The drawing under review shows one solid part. Ordinate dimensions are in mm from its lowest x, y, z. A direction names the side the tool comes from. Coordinates: 2 decimals unless noted, no trailing zeros. Write each loop counter-clockwise with the first axis right and the second up, starting at its lowest first coordinate (ties: lowest second). Pieces come first, ordered by that corner, then holes. Notation, with made-up numbers: M -20.75,69.25 L -9.75,69.25 A22 ccw -9.75,78.25 Z; hole C 49.5,75.25 d1. An arc over 180 degrees is marked long. Write item = value, one per line.
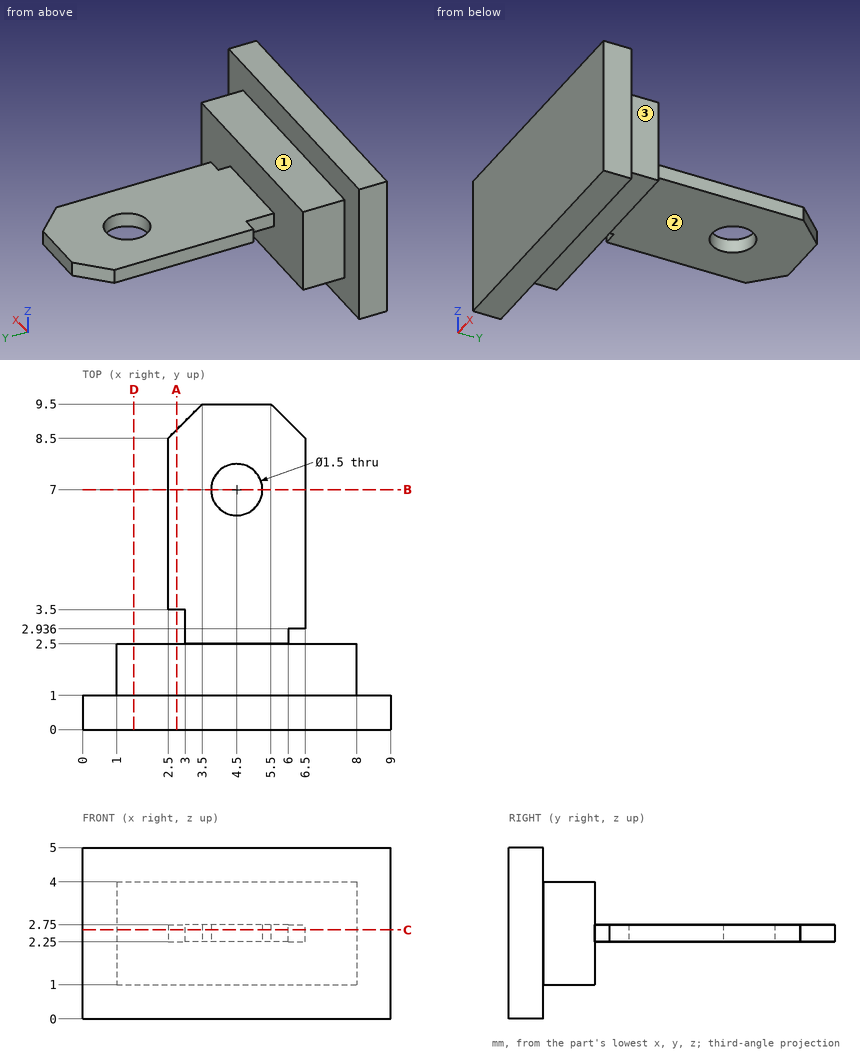
Q1. For P1, Ø4, axis at x = 7.5, y = 3.5, coming from the +Z side; P2, Ø1.2, axis at y = 2, z = 2, coming from the +X side; P3, Ø1.6, axis at x = 6, y = 2, coming from the -Z side, all flat-tipped, find the tip position at first contact; note any pin that passes through.
Check result:
P1 = 4
P2 = 8
P3 = 1
Q2. Consider section A-A, the plane x = 2.75. State the section outline as (y, z) points.
Check result:
outline = M 0,0 L 1,0 L 1,1 L 2.5,1 L 2.5,4 L 1,4 L 1,5 L 0,5 Z; M 3.5,2.25 L 8.75,2.25 L 8.75,2.75 L 3.5,2.75 Z
Q3. Wall thickness on line 1 (Y direction, x = 4.5, z = 2.45); line 2 (Y direction, x = 7.75, z = 0.75); line 3 (Y direction, x = 3, z = 3.4): over which ranges is each line inside the solid? List them lowest first.
Check result:
line_1 = 0 to 6.25, 7.75 to 9.5
line_2 = 0 to 1
line_3 = 0 to 2.5
Q4. Machinability: for the marked faces 1, 2 and 3, which of the approach directions +Z, -Z, +X, -X, +Y, -Y give a long, thin tool a straight path to every point of the face, cutting with its end or side? Answer none if there is none.
Check result:
face_1 = +Z, +X, -X, +Y
face_2 = -Z, +X, -X, +Y
face_3 = +Z, -Z, +X, +Y
Q5. Consider section D-D, the plane x = 1.5. State the section outline as (y, z) points.
Check result:
outline = M 0,0 L 1,0 L 1,1 L 2.5,1 L 2.5,4 L 1,4 L 1,5 L 0,5 Z
Q6. Consider section B-B, the plane y = 7. State the section outline as (x, z) points.
Check result:
outline = M 2.5,2.25 L 3.75,2.25 L 3.75,2.75 L 2.5,2.75 Z; M 5.25,2.25 L 6.5,2.25 L 6.5,2.75 L 5.25,2.75 Z
Q7. Consider section C-C, the plane z = 2.6. State the section outline as (x, y) points.
Check result:
outline = M 0,0 L 9,0 L 9,1 L 8,1 L 8,2.5 L 6,2.5 L 6,2.94 L 6.5,2.94 L 6.5,8.5 L 5.5,9.5 L 3.5,9.5 L 2.5,8.5 L 2.5,3.5 L 3,3.5 L 3,2.5 L 1,2.5 L 1,1 L 0,1 Z; hole C 4.5,7 d1.5
